The model under review builds one solid part; all positions refer to its coordinate system, in mm. A direction names the side the tool comes from. Coordinates: 2 decimals unless noted, no trailing zeros. Order: outer loops, then holes, each group sorted by start corner. A loop starts at its lowest first (then second) coordinate and runs counter-clockwise, first axis right, second up. Notation, with made-up numbers: (62.5, -21) - (71.5, -21) arc R23 cw to (71.5, 17) - close; hole circle Ø7 at (12.25, 63.5). An arc over 180 degrees is marked (long way). Answer in a Markdown table with one row per item.
```python
from build123d import *

# Parameters (mm, degrees)
SKETCH1_W              = 9.5
SKETCH1_H              = 4
BOSS_EXTRUDE1_DEPTH    = 10.5
BREAKBEAM_HOLE_1_DEPTH = 9.5
SKETCH5_W              = 4
SKETCH5_H              = 10.5
BOSS_EXTRUDE4_DEPTH    = 2.5
FILLET1_R              = 1
M2_CLEARANCE_HOLE_D    = 2.2
SKETCH15_W             = 7.7
SKETCH15_H             = 10.1
SKETCH15_W_2           = 7.1
SKETCH15_H_2           = 9.5
CUT_EXTRUDE5_DEPTH     = 2.544836551
CUT_EXTRUDE6_DEPTH     = 1.46


with BuildPart() as part:
    # Sketch1 → Boss-Extrude1 (new body)
    with BuildSketch(Plane(origin=(0, 0, 0), x_dir=(1, 0, 0), z_dir=(0, 1, 0))):
        with Locations((4.75, -2)):
            Rectangle(SKETCH1_W, SKETCH1_H)
    extrude(amount=BOSS_EXTRUDE1_DEPTH)

    # Sketch2 → Breakbeam Hole 1 (cut)
    with BuildSketch(Plane(origin=(0, 10.5, 0), x_dir=(1, 0, 0), z_dir=(0, 1, 0))):
        Polygon((8.25, -2.544836551), (8.25, -1.5), (8.25, 0), (1.15, 0), (1.15, -1.5), (1.15, -2.544836551), align=None)
    extrude(amount=-BREAKBEAM_HOLE_1_DEPTH, mode=Mode.SUBTRACT)

    # Sketch5 → Boss-Extrude4 (add)
    with BuildSketch(Plane.ZY):
        with Locations((2, 5.25)):
            Rectangle(SKETCH5_W, SKETCH5_H)
    extrude(amount=BOSS_EXTRUDE4_DEPTH)

    # Fillet1
    fillet1_edges = [part.edges().sort_by_distance(p)[0] for p in [
        (9.5, 10.5, 2),
        (-2.5, 0, 2),
        (-2.5, 10.5, 2),
        (9.5, 0, 2),
    ]]
    fillet(fillet1_edges, radius=FILLET1_R)

    # M2 Clearance Hole (through all)
    with Locations(Plane.XY.offset(4)):
        with Locations((-0.6, 8), (-0.6, 2.5)):
            Hole(M2_CLEARANCE_HOLE_D / 2)

    # Sketch15 → Cut-Extrude5 (cut)
    with BuildSketch(Plane(origin=(0, 0, 0), x_dir=(-1, 0, 0), z_dir=(0, 0, -1))):
        with Locations((-4.7, 5.75)):
            Rectangle(SKETCH15_W, SKETCH15_H)
        with Locations((-4.7, 5.75)):
            Rectangle(SKETCH15_W_2, SKETCH15_H_2, mode=Mode.SUBTRACT)
    extrude(amount=-CUT_EXTRUDE5_DEPTH, mode=Mode.SUBTRACT)

    # Sketch16 → Cut-Extrude6 (cut)
    with BuildSketch(Plane.XY.offset(4)):
        with BuildLine():
            Line((3.45, 5.9), (5.95, 5.9))
            ThreePointArc((5.95, 5.9), (7.1, 4.75), (5.95, 3.6))
            Line((5.95, 3.6), (3.45, 3.6))
            ThreePointArc((3.45, 3.6), (2.3, 4.75), (3.45, 5.9))
        make_face()
    extrude(amount=-CUT_EXTRUDE6_DEPTH, mode=Mode.SUBTRACT)


solid = part.part
```
Item 1: We need section D-D, the plane x = 5.5. Write out the cut boundary in (y, z).
Check values:
| item | result |
|---|---|
| outline | (0, 0) - (0.7, 0) - (0.7, 2.54) - (3.6, 2.54) - (3.6, 4) - (0, 4) - close; (5.9, 2.54) - (10.5, 2.54) - (10.5, 4) - (5.9, 4) - close |
Item 2: Mouldability with a two-part tool opening along X and no side actions: class faces 4 (the face through (5, 7, 2.545)), 5 (the face through (0, 4, 0)), 6 (the face through (-2.199, 10.215, 2.028)) as +X half, -X half, draft (parallel to the pull), parting line (faces both ways), or undercut.
Check values:
| item | result |
|---|---|
| face 4 | undercut |
| face 5 | draft |
| face 6 | -X half |
Item 3: Tool access review of faces 1 (the face through (5, 5.9, 3)), 2 (the face through (-2.199, 0.285, 2.028)), 3 (the face through (0.85, 6, 1)): name each direction out of +Z, -Z, +X, -X, +Y, -Y from which nothing blocks a thin tool from reaching the whole face with its end or side.
Check values:
| item | result |
|---|---|
| face 1 | +Z, -Z |
| face 2 | +Z, -Z, -X, -Y |
| face 3 | -Z, +Y |
Item 4: To check wall thickness, follow line 1 (Y direction, x = -0.6, z = 2.5); line 2 (X direction, y = 1, z = 1.35); line 3 (Y direction, x = 0, z = 0.65). State the ranges of each line that lie inside material, in increasing order. Write a range as from..to.
Check values:
| item | result |
|---|---|
| line 1 | 0..1.4, 3.6..6.9, 9.1..10.5 |
| line 2 | -2.5..0.85, 8.55..9.5 |
| line 3 | 0..1.58, 3.42..7.08, 8.92..10.5 |
Item 5: We need section C-C, the plane y = 2.5. Write out the cut boundary in (x, z).
Check values:
| item | result |
|---|---|
| outline | (-2.5, 0) - (-1.7, 0) - (-1.7, 4) - (-2.5, 4) - close; (0.5, 0) - (0.85, 0) - (0.85, 2.54) - (8.55, 2.54) - (8.55, 0) - (9.5, 0) - (9.5, 4) - (0.5, 4) - close |
Item 6: Clearance check with flat-ended pins moving along their axes: pin 1 Ø4 at (x, y) = (5.5, 7.5) entering from -Z; pin 2 Ø2 at (x, z) = (6, 1) entering from +Y. State where each tip first meets the part, or that it passes through.
Check values:
| item | result |
|---|---|
| pin 1 | z = 2.54 |
| pin 2 | y = 0.7 |
Item 7: We need section B-B, the plane z = 3.7. Write out the cut boundary in (x, y), then the cut area to 3 significant figures.
Check values:
| item | result |
|---|---|
| outline | (-2.5, 1) arc R1 ccw to (-1.5, 0) - (8.5, 0) arc R1 ccw to (9.5, 1) - (9.5, 9.5) arc R1 ccw to (8.5, 10.5) - (-1.5, 10.5) arc R1 ccw to (-2.5, 9.5) - close; hole circle Ø2.2 at (-0.6, 2.5); hole circle Ø2.2 at (-0.6, 8); hole (3.45, 3.6) - (5.95, 3.6) arc R1.15 ccw to (5.95, 5.9) - (3.45, 5.9) arc R1.15 ccw to start |
| area | 108 mm^2 |
Item 8: We need section A-A, the plane x = -0.6. Write out the cut boundary in (y, z), then the cut area to 3 significant figures.
Check values:
| item | result |
|---|---|
| outline | (0, 0) - (1.4, 0) - (1.4, 4) - (0, 4) - close; (3.6, 0) - (6.9, 0) - (6.9, 4) - (3.6, 4) - close; (9.1, 0) - (10.5, 0) - (10.5, 4) - (9.1, 4) - close |
| area | 24.4 mm^2 |
